The listing builds one solid part. Answer for the finished solid, in the listing's coordinates (mm). Face numbers are marked on the shaded views. Coordinates: 2 decimals unless noted, no trailing zeros. Order: outer loops, then holes, each group sorted by start corner. A loop starts at its lowest first (then second) coordinate and runs counter-clockwise, first axis right, second up.
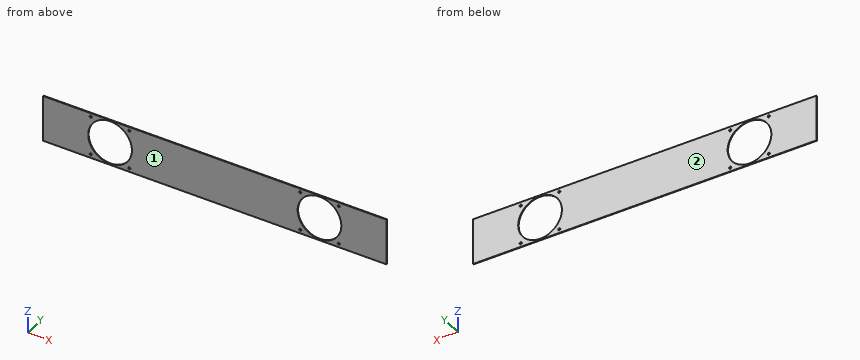
from build123d import *

# Parameters (mm, degrees)
F0_W     = 935
F0_H     = 125
F0_R     = 3
F0_R_2   = 59.5
F1_DEPTH = 2


with BuildPart() as f1:
    # F0 (on Front) → F1 (new body)
    with BuildSketch(Plane.XZ):
        with Locations((336.224301, -21.191215)):
            Rectangle(F0_W, F0_H)
        with Locations((-1.490244, -73.691215)):
            Circle(F0_R, mode=Mode.SUBTRACT)
        with Locations((103.757686, -73.691215)):
            Circle(F0_R, mode=Mode.SUBTRACT)
        with Locations((568.724301, -73.691215)):
            Circle(F0_R, mode=Mode.SUBTRACT)
        with Locations((673.724301, -73.691215)):
            Circle(F0_R, mode=Mode.SUBTRACT)
        with Locations((51.257686, -21.191215)):
            Circle(F0_R_2, mode=Mode.SUBTRACT)
        with Locations((-1.242314, 31.308785)):
            Circle(F0_R, mode=Mode.SUBTRACT)
        with Locations((103.757686, 31.308785)):
            Circle(F0_R, mode=Mode.SUBTRACT)
        with Locations((621.224301, -21.191215)):
            Circle(F0_R_2, mode=Mode.SUBTRACT)
        with Locations((568.724301, 31.308785)):
            Circle(F0_R, mode=Mode.SUBTRACT)
        with Locations((673.724301, 31.308785)):
            Circle(F0_R, mode=Mode.SUBTRACT)
    extrude(amount=F1_DEPTH)


solid = f1.part
(1) Find section D-D on z = 2. Determine the outline of the cut face in (x, y).
(2) Given pin 1 Ø3.5 at (x, z) = (-1.49, -73.69) entering from -Y, flat-ended and moving along its own axis, determine where the tip first touches the part or whether it passes through.
(3) Find section C-C on y = -0.9. Count the separate pieces of the cut face and the enclosed holes in it, then the cut area to 3 significant figures.
(4) The mould has two halves that part along Y. Classify the marked faces 1 and 2: pulls with the +Y half, pulls with the -Y half, needs draft (parallel to the pull), parting line crosses it, or undercut.
(5) Find section B-B on x = 79. Determine the outline of the cut face in (y, z), then the cut area to 3 significant figures.
(6) Find the intervals of material crossed by probe 1 along X at (y, z) = (-1.1, -54); probe 2 along X at (y, z) = (-1.8, 20), in increasing order.
(7) Find section A-A on z = -50.5. Determine the outline of the cut face in (x, y), then the cut area to 3 significant figures.
Resolved:
1. outline: (-131.28, -2) - (-3.54, -2) - (-3.54, 0) - (-131.28, 0) - close; (106.05, -2) - (566.43, -2) - (566.43, 0) - (106.05, 0) - close; (676.02, -2) - (803.72, -2) - (803.72, 0) - (676.02, 0) - close
2. pin 1: passes through
3. separate pieces: 1
3. enclosed holes: 10
3. area: 94,400 mm2
4. face 1: pulls with the -Y half
4. face 2: pulls with the +Y half
5. outline: (-2, -83.69) - (0, -83.69) - (0, -73.83) - (-2, -73.83) - close; (-2, 31.45) - (0, 31.45) - (0, 41.31) - (-2, 41.31) - close
5. area: 39.5 mm2
6. probe 1: x = -131.28 to 1.62, 100.89 to 571.59, 670.86 to 803.72
6. probe 2: x = -131.28 to 8.32, 94.19 to 578.29, 664.16 to 803.72
7. outline: (-131.28, -2) - (-0.52, -2) - (-0.52, 0) - (-131.28, 0) - close; (103.04, -2) - (569.44, -2) - (569.44, 0) - (103.04, 0) - close; (673.01, -2) - (803.72, -2) - (803.72, 0) - (673.01, 0) - close
7. area: 1,460 mm2
